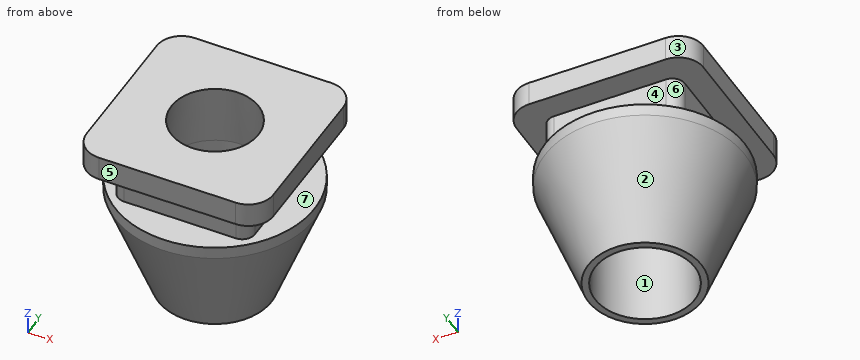
from build123d import *
from build123d.topology import SkipClean

# Parameters (mm, degrees)
SKETCH1_W           = 15
SKETCH1_H           = 15
SKETCH1_R           = 4
BOSS_EXTRUDE1_DEPTH = 2
BOSS_EXTRUDE2_START = 3.2
SKETCH2_W           = 11
SKETCH2_H           = 11
SKETCH2_R           = 4
BOSS_EXTRUDE2_DEPTH = 3.2
BOSS_EXTRUDE3_START = 10
SKETCH3_R           = 8
SKETCH3_R_2         = 4
BOSS_EXTRUDE3_DEPTH = 10
CHAMFER1_SIZE       = 9
CHAMFER1_SIZE2      = 3.454776315
FILLET1_R           = 2
FILLET2_R           = 1


with BuildPart() as part:
    # Sketch1 → Boss-Extrude1 (new body)
    with BuildSketch(Plane.XY):
        Rectangle(SKETCH1_W, SKETCH1_H)
        Circle(SKETCH1_R, mode=Mode.SUBTRACT)
    extrude(amount=BOSS_EXTRUDE1_DEPTH)

    # Sketch2 → Boss-Extrude2 (add)
    with SkipClean():  # the faces are left unmerged after this step: merging them gives an invalid solid
        with BuildSketch(Plane(origin=(0, 0, 0), x_dir=(-1, 0, 0), z_dir=(0, 0, -1)).offset(BOSS_EXTRUDE2_START)):
            Rectangle(SKETCH2_W, SKETCH2_H)
            Circle(SKETCH2_R, mode=Mode.SUBTRACT)
        extrude(amount=-BOSS_EXTRUDE2_DEPTH)

    # Sketch3 → Boss-Extrude3 (add)
    with SkipClean():  # the faces are left unmerged after this step: merging them gives an invalid solid
        with BuildSketch(Plane(origin=(0, 0, -3.2), x_dir=(-1, 0, 0), z_dir=(0, 0, -1)).offset(BOSS_EXTRUDE3_START)):
            Circle(SKETCH3_R)
            Circle(SKETCH3_R_2, mode=Mode.SUBTRACT)
        extrude(amount=-BOSS_EXTRUDE3_DEPTH)

    # Sketch4 → Revolve1 (revolve)
    with BuildSketch(Plane(origin=(0, 0, 0), x_dir=(1, 0, 0), z_dir=(0, 1, 0))):
        Polygon((-4, -2), (-3.5, -2), (-4, 3.2), align=None)
    revolve(axis=Axis((0, 0, -13.2), (0, 0, 1)))

    # Chamfer1
    chamfer1_edges = [part.edges().sort_by_distance(p)[0] for p in [
        (8, 0, -13.2),
    ]]
    chamfer1_side = [part.faces().sort_by_distance(p)[0] for p in [
        (8, 0, -8.2),
    ]]
    chamfer(chamfer1_edges, length=CHAMFER1_SIZE, length2=CHAMFER1_SIZE2, reference=chamfer1_side[0])

    # Fillet1
    fillet1_edges = [part.edges().sort_by_distance(p)[0] for p in [
        (7.5, -7.5, 1),
        (-7.5, -7.5, 1),
        (-7.5, 7.5, 1),
        (7.5, 7.5, 1),
    ]]
    fillet(fillet1_edges, radius=FILLET1_R)

    # Fillet2
    fillet2_edges = [part.edges().sort_by_distance(p)[0] for p in [
        (-5.5, -5.5, -1.6),
        (-5.5, 5.5, -1.6),
        (5.5, 5.5, -1.6),
        (5.5, -5.5, -1.6),
    ]]
    fillet(fillet2_edges, radius=FILLET2_R)


solid = part.part
Model file for the job. Use its own axes, mm. Face numbers are marked on the shaded views. A direction names the side the tool comes from. Give positions to 0.01 mm unless a question says otherwise; leave off trailing zeros. Order: outer loops, then holes, each group sorted by start corner. A loop starts at its lowest first (then second) coordinate and runs counter-clockwise, first axis right, second up. Notation, with made-up numbers: M 2.25,4.25 L 17.25,4.25 A17 cw 17.25,15.25 Z; hole C 7.25,52.25 d2. An arc over 180 degrees is marked long. Write item = value, one per line.
Q1. Tool access for the marked faces 4, 5, 6 and 7: list every direction of +Z, -Z, +X, -X, +Y, -Y with a clear straight run to the whole face (end or side of a thin tool).
Derived:
face_4 = +X, -X, +Y
face_5 = +Z, +X, -X, -Y
face_6 = -X, +Y
face_7 = none
Q2. Cut at C-C, the plane z = -0.25. List the corners of the cut face in (x, y).
Derived:
outline = M -5.5,-4.5 A1 ccw -4.5,-5.5 L 4.5,-5.5 A1 ccw 5.5,-4.5 L 5.5,4.5 A1 ccw 4.5,5.5 L -4.5,5.5 A1 ccw -5.5,4.5 Z; hole C 0,0 d7.43
Q3. Drill centre lines: line 1 (Z direction, x = 6.75, y = 4.5); line 2 (X direction, y = 1.25, z = -1); line 3 (X direction, y = -1.75, z = -9.75). Where is each one in solid material? Low to high. Write a range as [from, to].
Derived:
line_1 = [0, 2]
line_2 = [-5.5, -3.58], [3.58, 5.5]
line_3 = [-5.6, -3.6], [3.6, 5.6]
Q4. Cut at A-A, the plane y = 0. List the corners of the cut face in (x, z), then the cut area to 3 significant figures.
Derived:
outline = M -8,-4.2 L -4.55,-13.2 L -4,-13.2 L -4,-3.2 L -3.5,2 L -7.5,2 L -7.5,0 L -5.5,0 L -5.5,-3.2 L -8,-3.2 Z; M 3.5,2 L 4,-3.2 L 4,-13.2 L 4.55,-13.2 L 8,-4.2 L 8,-3.2 L 5.5,-3.2 L 5.5,0 L 7.5,0 L 7.5,2 Z
area = 75.1 mm2
Q5. Two-plate mould, pull along X, no slides. Class the marked faces 1, 2 and 3: pulls with the +X half, pulls with the -X half, needs draft (parallel to the pull), parting line crosses it, or undercut.
Derived:
face_1 = undercut
face_2 = parting line crosses it
face_3 = pulls with the -X half
Q6. Cut at D-D, the plane z = -2. List the corners of the cut face in (x, y).
Derived:
outline = M -5.5,-4.5 A1 ccw -4.5,-5.5 L 4.5,-5.5 A1 ccw 5.5,-4.5 L 5.5,4.5 A1 ccw 4.5,5.5 L -4.5,5.5 A1 ccw -5.5,4.5 Z; hole C 0,0 d7.77
Q7. Flat gauge pins, fed straight in: pin 1 (1 mm diameter, centred on x = -6, z = -6, fed in from +Y); pin 2 (1.5 mm diameter, centred on x = -2, z = -3, fed in from -Y); pin 3 (5 mm diameter, centred on y = 1, z = -8.5, fed in from +X). Where does each tip first touch, or does it go through?
Derived:
pin_1 = 4.88
pin_2 = -7.9
pin_3 = 7.27
